Source: CAD feature listing. Evaluate the final solid. Frame: model axes, mm. A direction names the side the tool comes from. Round coordinates to 2 decimals unless told otherwise and drop trailing zeros. Loops run counter-clockwise (first coordinate to the right, second up) from the corner with the lowest first, then second, coordinate; pieces in that order, holes last.
(1) Section B-B, the plane y = -30.5. Return the cut outline in (x, z).
(2) Set-up query: faces 4 (the cylindrical face through (-56.26, -38.42, 4.14)), 5 (the cylindrical face through (47.22, -41.11, 11.45)). Return all of +Z, -Z, +X, -X, +Y, -Y with unobstructed straight access to the full face (end or side cutting, diameter ignored); none if empty.
(3) Section A-A, the plane z = 4. Return the cut outline in (x, y), plus the area to 3 significant figures.
(4) Material intervals for probe 1 along Y at (x, z) = (-57, 5.65); probe 2 along X at (y, z) = (14, 4.75); probe 3 along X at (y, z) = (-7, 8.75), sorted ascending.
(5) Section D-D, the plane x = 26. Return the cut outline in (y, z).
(6) Mould query, pull axis Y, two halves, no side actions, for faces 1 (the flat face through (-5, 39, 6.6)), 2 (the flat face through (-1, 1, 0)), 3 (the flat face through (-1, 41.9, 7)). Classes: pulls with the +Y half, pulls with the -Y half, needs draft (parallel to the pull), parting line crosses it, or undercut.
(7) First-contact query: pin 1 Ø2 at (x, y) = (-40.5, 18) entering from +Z; pin 2 Ø0.5 at (x, y) = (47.5, 41) entering from +Z. Flat tips, straight axial feed; report the tip coordinate or a pass-through.
(8) Section C-C, the plane x = 57. Return the cut outline in (y, z).
```python
from build123d import *

# Parameters (mm, degrees)
SKETCH1_W            = 120.6
SKETCH1_H            = 80.6
BOSS_EXTRUDE1_DEPTH  = 1.6
SKETCH2_W            = 123.8
SKETCH2_H            = 83.8
SKETCH2_W_2          = 120.6
SKETCH2_H_2          = 80.6
BOSS_EXTRUDE2_DEPTH  = 8.2
SKETCH3_W            = 120.6
SKETCH3_H            = 80.6
BOSS_EXTRUDE3_DEPTH  = 5
SKETCH4_R            = 1.6
CUT_EXTRUDE1_DEPTH   = 5
SKETCH5_W            = 40.4
SKETCH5_H            = 1.6
SKETCH5_W_2          = 6.6
BOSS_EXTRUDE4_DEPTH  = 6.8
SKETCH6_R            = 3.55
CUT_EXTRUDE2_DEPTH   = 6.8
BOSS_EXTRUDE5_DEPTH  = 6.8
SKETCH8_W            = 1.6
SKETCH8_H            = 37
BOSS_EXTRUDE6_DEPTH  = 2.2
SKETCH9_W            = 30.6
SKETCH9_H            = 1.6
SKETCH9_W_2          = 2.8
BOSS_EXTRUDE7_DEPTH  = 6.8
CUT_EXTRUDE3_DEPTH   = 6.8
SKETCH11_W           = 15
SKETCH11_H           = 1.6
BOSS_EXTRUDE8_DEPTH  = 6.8
SKETCH12_W           = 8.4
SKETCH12_H           = 3.4
CUT_EXTRUDE4_DEPTH   = 6.8
BOSS_EXTRUDE9_DEPTH  = 6.8
SKETCH14_W           = 62.6
SKETCH14_H           = 1.6
BOSS_EXTRUDE10_DEPTH = 1.2


with BuildPart() as part:
    # Sketch1 → Boss-Extrude1 (new body)
    with BuildSketch(Plane.XY):
        Rectangle(SKETCH1_W, SKETCH1_H)
    extrude(amount=BOSS_EXTRUDE1_DEPTH)

    # Sketch2 → Boss-Extrude2 (add)
    with BuildSketch(Plane.XY):
        Rectangle(SKETCH2_W, SKETCH2_H)
        Rectangle(SKETCH2_W_2, SKETCH2_H_2, mode=Mode.SUBTRACT)
    extrude(amount=BOSS_EXTRUDE2_DEPTH)

    # Sketch3 → Boss-Extrude3 (add)
    with BuildSketch(Plane.XY.offset(1.6)):
        Rectangle(SKETCH3_W, SKETCH3_H)
        Polygon((-58.7, 34.3), (-54.3, 34.3), (-54.3, 38.5), (54.3, 38.5), (54.3, 34.3), (58.7, 34.3), (58.7, -34.3), (54.3, -34.3), (54.3, -38.7), (-54.3, -38.7), (-54.3, -34.3), (-58.7, -34.3), align=None, mode=Mode.SUBTRACT)
    extrude(amount=BOSS_EXTRUDE3_DEPTH)

    # Sketch4 → Cut-Extrude1 (cut)
    with BuildSketch(Plane.XY.offset(6.6)):
        with Locations((-57, 37)):
            Circle(SKETCH4_R)
        with Locations((57, 37)):
            Circle(SKETCH4_R)
        with Locations((57, -37)):
            Circle(SKETCH4_R)
        with Locations((-57, -37)):
            Circle(SKETCH4_R)
    extrude(amount=-CUT_EXTRUDE1_DEPTH, mode=Mode.SUBTRACT)

    # Sketch5 → Boss-Extrude4 (add)
    with BuildSketch(Plane.XY.offset(8.2)):
        with Locations((41.7, -41.1)):
            Rectangle(SKETCH5_W, SKETCH5_H)
        with Locations((10.6, -41.1)):
            Rectangle(SKETCH5_W_2, SKETCH5_H)
    extrude(amount=BOSS_EXTRUDE4_DEPTH)

    # Sketch6 → Cut-Extrude2 (cut)
    with BuildSketch(Plane.XZ.offset(41.9)):
        with Locations((32.1, 15)):
            Circle(SKETCH6_R)
        with Locations((47.3, 15)):
            Circle(SKETCH6_R)
    extrude(amount=-CUT_EXTRUDE2_DEPTH, mode=Mode.SUBTRACT)

    # Sketch7 → Boss-Extrude5 (add)
    with BuildSketch(Plane.XY.offset(8.2)):
        Polygon((-61.9, -26.1), (-61.9, -41.9), (-55.3, -41.9), (-55.3, -40.3), (-60.3, -40.3), (-60.3, -26.1), align=None)
    extrude(amount=BOSS_EXTRUDE5_DEPTH)

    # Sketch8 → Boss-Extrude6 (add)
    with BuildSketch(Plane.XY.offset(8.2)):
        with Locations((-61.1, -7.6)):
            Rectangle(SKETCH8_W, SKETCH8_H)
    extrude(amount=BOSS_EXTRUDE6_DEPTH)

    # Sketch9 → Boss-Extrude7 (add)
    with BuildSketch(Plane.XY.offset(8.2)):
        Polygon((-60.3, 35.8), (-61.9, 35.8), (-61.9, 41.9), (-34.3, 41.9), (-34.3, 40.3), (-60.3, 40.3), align=None)
        with Locations((-11.4, 41.1)):
            Rectangle(SKETCH9_W, SKETCH9_H)
        with Locations((12.9, 41.1)):
            Rectangle(SKETCH9_W_2, SKETCH9_H)
    extrude(amount=BOSS_EXTRUDE7_DEPTH)

    # Sketch10 → Cut-Extrude3 (cut)
    with BuildSketch(Plane(origin=(0, 41.9, 0), x_dir=(1, 0, 0), z_dir=(0, 1, 0))):
        with BuildLine():
            Line((-45.35, -12.4), (-45.35, -15))
            Line((-45.35, -15), (-40.85, -15))
            Line((-40.85, -15), (-40.85, -12.4))
            ThreePointArc((-40.85, -12.4), (-43.1, -10.15), (-45.35, -12.4))
        make_face()
    extrude(amount=-CUT_EXTRUDE3_DEPTH, mode=Mode.SUBTRACT)

    # Sketch11 → Boss-Extrude8 (add)
    with BuildSketch(Plane.XY.offset(8.2)):
        with Locations((31.3, 41.1)):
            Rectangle(SKETCH11_W, SKETCH11_H)
    extrude(amount=BOSS_EXTRUDE8_DEPTH)

    # Sketch12 → Cut-Extrude4 (cut)
    with BuildSketch(Plane(origin=(0, 41.9, 0), x_dir=(1, 0, 0), z_dir=(0, 1, 0))):
        with Locations((32, -13.3)):
            Rectangle(SKETCH12_W, SKETCH12_H)
    extrude(amount=-CUT_EXTRUDE4_DEPTH, mode=Mode.SUBTRACT)

    # Sketch13 → Boss-Extrude9 (add)
    with BuildSketch(Plane.XY.offset(8.2)):
        Polygon((61.9, -40.3), (60.3, -40.3), (60.3, 40.3), (53.1, 40.3), (53.1, 41.9), (61.9, 41.9), align=None)
    extrude(amount=BOSS_EXTRUDE9_DEPTH)

    # Sketch14 → Boss-Extrude10 (add)
    with BuildSketch(Plane.XY.offset(8.2)):
        with Locations((-24, -41.1)):
            Rectangle(SKETCH14_W, SKETCH14_H)
    extrude(amount=BOSS_EXTRUDE10_DEPTH)


solid = part.part
```
Output values:
1. outline: (-61.9, 0) - (61.9, 0) - (61.9, 15) - (60.3, 15) - (60.3, 6.6) - (58.7, 6.6) - (58.7, 1.6) - (-58.7, 1.6) - (-58.7, 6.6) - (-60.3, 6.6) - (-60.3, 15) - (-61.9, 15) - close
2. face 4: +Z
2. face 5: +Z, +Y, -Y
3. outline: (-61.9, -41.9) - (61.9, -41.9) - (61.9, 41.9) - (-61.9, 41.9) - close; hole (-58.7, -34.3) - (-54.3, -34.3) - (-54.3, -38.7) - (54.3, -38.7) - (54.3, -34.3) - (58.7, -34.3) - (58.7, 34.3) - (54.3, 34.3) - (54.3, 38.5) - (-54.3, 38.5) - (-54.3, 34.3) - (-58.7, 34.3) - close; hole circle Ø3.2 at (-57, -37); hole circle Ø3.2 at (-57, 37); hole circle Ø3.2 at (57, -37); hole circle Ø3.2 at (57, 37)
3. area: 1,350 mm2
4. probe 1: y = -41.9 to -38.6, -35.4 to -34.3, 34.3 to 35.4, 38.6 to 41.9
4. probe 2: x = -61.9 to -58.7, 58.7 to 61.9
4. probe 3: x = -61.9 to -60.3, 60.3 to 61.9
5. outline: (-41.9, 0) - (41.9, 0) - (41.9, 15) - (40.3, 15) - (40.3, 6.6) - (38.5, 6.6) - (38.5, 1.6) - (-38.7, 1.6) - (-38.7, 6.6) - (-40.3, 6.6) - (-40.3, 15) - (-41.9, 15) - close
6. face 1: undercut
6. face 2: needs draft
6. face 3: pulls with the +Y half
7. pin 1: stops at z = 1.6
7. pin 2: stops at z = 8.2
8. outline: (-41.9, 0) - (41.9, 0) - (41.9, 15) - (40.3, 15) - (40.3, 6.6) - (38.6, 6.6) - (38.6, 1.6) - (35.4, 1.6) - (35.4, 6.6) - (34.3, 6.6) - (34.3, 1.6) - (-34.3, 1.6) - (-34.3, 6.6) - (-35.4, 6.6) - (-35.4, 1.6) - (-38.6, 1.6) - (-38.6, 6.6) - (-40.3, 6.6) - (-40.3, 15) - (-41.9, 15) - close
